For this review, use the dimensioned drawing (mm, ordinates from the lowest corner) and the shaded views. A direction names the side the tool comes from. Round coordinates to 2 decimals unless told otherwise and drop trailing zeros. Write each loop counter-clockwise with the first axis right and the second up, starting at its lowest first coordinate (ties: lowest second). Pieces come first, ordered by that corner, then holes. Notation, with made-up numbers: (85, 73.25) - (121, 73.25) arc R29 ccw to (121, 111.25) - close; hole circle Ø4 at (-9.5, 74.25). An arc over 180 degrees is marked (long way). Return JSON: item names as keys, results as strings.
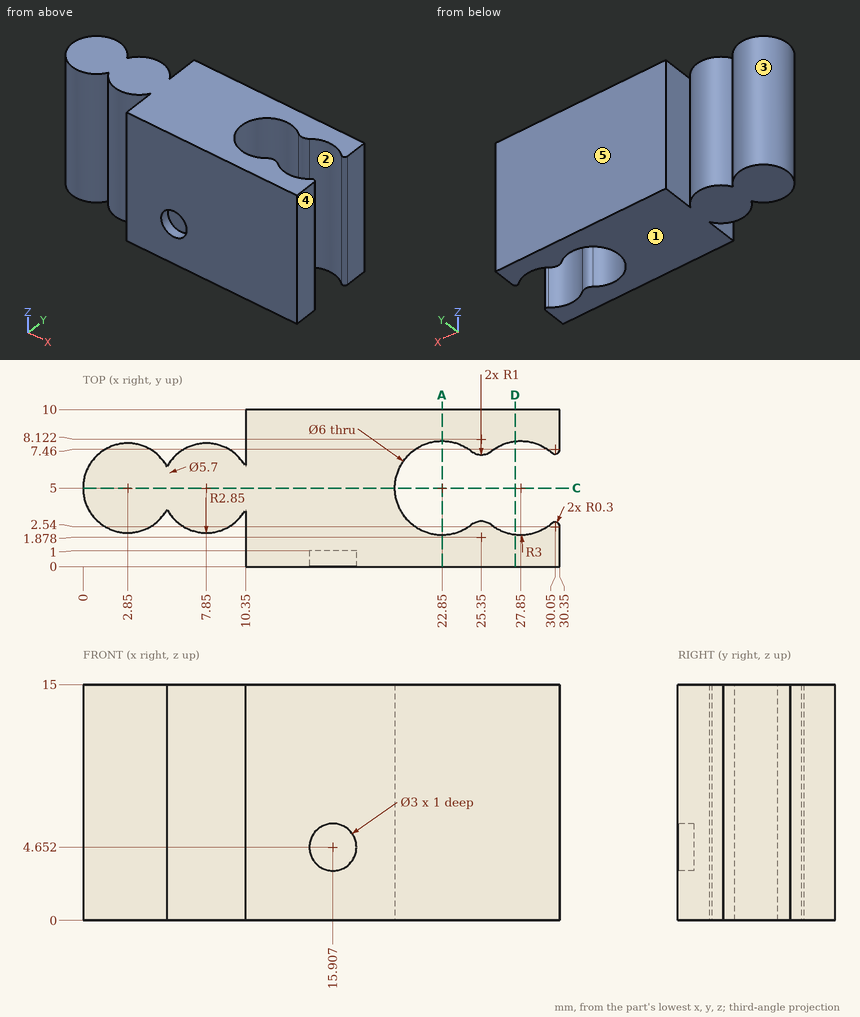
(1) For the marked faces 1 and 2, list the 3-axis set-ups (+Z, -Z, +X, -X, +Y, -Y) from which the entire face can be reached by the end or side of a thin tool; tool diameter is ignored.
Filled in:
{"face 1": "-Z, +X, -X, +Y, -Y", "face 2": "+Z, -Z"}
(2) Wall thickness on line 1 (Y direction, x = 25.5, z = 6) (1 decimal); line 2 (Y direction, x = 27.5, z = 0.75); line 3 (X direction, y = 8.5, z = 3): over which ranges is each line inside the solid? List them lowest first.
Filled in:
{"line 1": "y = 0 to 2.9, 7.1 to 10", "line 2": "y = 0 to 2.02, 7.98 to 10", "line 3": "x = 10.35 to 30.35"}
(3) Add section C-C (y = 5). Write out the cut boundary in (x, z), plus the area to 3 significant figures.
Filled in:
{"outline": "(0, 0) - (19.85, 0) - (19.85, 15) - (0, 15) - close", "area": "298 mm2"}
(4) Mouldability with a two-part tool opening along X and no side actions: class the marked faces 3, 4 and 5 as released by +X, released by -X, zero draft, split by the parting line, or undercut.
Filled in:
{"face 3": "undercut", "face 4": "released by +X", "face 5": "zero draft"}
(5) Add section A-A (x = 22.85). Write out the cut boundary in (y, z).
Filled in:
{"outline": "(0, 0) - (2, 0) - (2, 15) - (0, 15) - close; (8, 0) - (10, 0) - (10, 15) - (8, 15) - close"}
(6) Clearance check with flat-ended pins moving along their axes: pin 1 Ø2 at (y, z) = (3, 7.5) entering from -X; pin 2 Ø3 at (x, z) = (27, 10.5) entering from -Y; pin 3 Ø3 at (y, z) = (7, 10.5) entering from -X; pin 4 Ø1.8 at (y, z) = (2.5, 10.5) entering from -X. State where each tip first meets the part, or that it passes through.
Filled in:
{"pin 1": "stops at x = 0.18", "pin 2": "stops at y = 0", "pin 3": "stops at x = 0.04", "pin 4": "stops at x = 0.49"}
(7) Add section D-D (x = 27.5). Write out the cut boundary in (y, z).
Filled in:
{"outline": "(0, 0) - (2.02, 0) - (2.02, 15) - (0, 15) - close; (7.98, 0) - (10, 0) - (10, 15) - (7.98, 15) - close"}
